Read the model definition and answer for the solid it produces. Units are mm, in the model's axes. A direction names the side the tool comes from. Round coordinates to 2 decimals unless told otherwise and drop trailing zeros. Write each loop counter-clockwise with the first axis right and the second up, starting at its lowest first coordinate (ties: lowest second). Pieces come first, ordered by that corner, then holes. Notation, with made-up numbers: (44, 22.25) - (57, 22.25) arc R26 ccw to (57, 54.25) - close; hole circle Ø4 at (73, 49). An arc over 180 degrees is marked (long way). One line per item, written item: value. Start each with the question number.
(1) A cutting plane is placed at D-D, the plane z = 3. Determine the outline of the cut face in (x, y), plus the area to 3 significant figures.
(2) Find the intervals of material crossed by L1, parallel to X at y = -24.4, z = 16.7 (3 decimals); L2, parallel to Y at x = 15, z = 4.5; L3, parallel to Y at x = -22, z = -16, in increasing order.
(3) A cutting plane is placed at C-C, the plane x = 0. Determine the outline of the cut face in (y, z) (1 decimal).
(4) A cutting plane is placed at B-B, the plane y = 15. Determine the outline of the cut face in (x, z).
(5) A cutting plane is placed at A-A, the plane z = -8.7. Determine the outline of the cut face in (x, y) (1 decimal), plus the area to 3 significant figures.
(6) For faces 1 (the face through (0, -23.13, 21)), 2 (the face through (0, -23.13, -13)), 3 (the face through (-0.55, 24.994, 3.944)), determine the directions among +Z, -Z, +X, -X, +Y, -Y from which every point of the face is accessible in a straight line to the end or side of a thin tool.
(7) The mould has two halves that part along Z. Classify faces 4 (the face through (-17, -4, 8)), 5 (the face through (25, -19, 4)), 6 (the face through (-19.08, -25.6, -6.36)): +Z half, -Z half, draft (parallel to the pull), parting line (faces both ways), or undercut.
(8) Flat-ended cylindrical pins translate along their axes: pin 1 Ø17 at (x, z) = (7, 15.5) entering from +Y; pin 2 Ø6 at (x, z) = (8.5, 19) entering from +Y; pin 3 Ø6 at (x, y) = (14.5, -2.5) entering from +Z. Find the tip coordinate at first contact, or state that the pin passes through.
Autodesk Inventor part; units mm, degrees
ref_plane "YZ Plane" through (0, 0, 0) normal (1, 0, 0) x (0, 1, 0)
ref_plane "XZ Plane" through (0, 0, 0) normal (0, 1, 0) x (-1, 0, 0)
ref_plane "XY Plane" through (0, 0, 0) normal (0, 0, 1) x (1, 0, 0)
sketch "Sketch1" plane through (0, 0, 0) normal (0, 0, 1) x (1, 0, 0)
  circle A0 centre (0, 0) radius 17
  arc A1 (25, 0) -> (-25, 0) centre (0, 0) ccw
  line L0 (-25, 0) -> (-25, -23.1305)
  line L1 (-25, -23.1305) -> (25, -23.1305)
  line L2 (25, -23.1305) -> (25, 0)
  circle A2 centre (-15, 15) radius 2.25
  circle A3 centre (15, 15) radius 2.25
  circle A4 centre (-15, -15) radius 2.25
  circle A5 centre (15, -15) radius 2.25
  dimension "d0" = 34
  dimension "d1" = 50
  dimension "d2" = 50
  dimension "d3" = 23.1305
  dimension "d54" = 4.5
  dimension "d57" = 30
  dimension "d60" = 30
  dimension "d63" = 15
  dimension "d64" = 15
extrude "Extrusion1" add sketch "Sketch1" along normal blind 8 contours L2 L1 L0 A1 | A2 | A3 | A4 | A5
sketch "Sketch2" plane through (-25, -23.1305, 0) normal (0, -1, 0) x (1, 0, 0)
  line L0 (0, 0) -> (50, 0) construction
  line L1 (0, 0) -> (0, 8)
  line L2 (0, -21.4) -> (50, -21.4)
  line L3 (50, -21.4) -> (50, 29.4)
  line L4 (50, 29.4) -> (0, 29.4)
  line L5 (0, 29.4) -> (0, -21.4)
  line L6 (0, -21.4) -> (50, 29.4) construction
  line L7 (50, -21.4) -> (0, 29.4) construction
  point P0 (25, 0)
  point P1 (25, 4)
  point P2 (25, 4)
  point P3 (0, 4)
  point P4 (25, 4)
  point P5 (25, 0)
  point P6 (50, 8)
  dimension "d7" = 50.8
  dimension "d65" = 50
  dimension "d66" = 50
extrude "Extrusion2" add sketch "Sketch2" along normal blind 5
sketch "Sketch3" plane through (-25, -28.1305, 0) normal (0, -1, 0) x (1, 0, 0)
  line L0 (50, 29.4) -> (0, 29.4)
  line L1 (0, 29.4) -> (0, -21.4)
  point P0 (25, 0)
  point P1 (8.0667, 16.7)
  point P2 (25, 16.7)
  point P3 (8.0667, -8.7)
  point P4 (25, -8.7)
  point P5 (41.9333, 16.7)
  point P6 (41.9333, -8.7)
  dimension "d39" = 16.9333
  dimension "d42" = 25.4
  dimension "d45" = 12.7
  dimension "d67" = 50
  dimension "d68" = 50.8
  dimension "d70" = 8.0667
hole "Hole2" at (-16.9333, -28.1305, 16.7) at (0, -28.1305, 16.7) at (-16.9333, -28.1305, -8.7) at (0, -28.1305, -8.7) at (16.9333, -28.1305, 16.7) at (16.9333, -28.1305, -8.7) direction (0, 1, 0) diameter 6.35 end through all
sketch "Sketch4" plane through (0, 0, 0) normal (0, 0, -1) x (-1, 0, 0)
  circle A0 centre (0, 0) radius 17
  line L0 (25, 0) -> (25, -23.1305)
  line L1 (25, -23.1305) -> (-25, -23.1305)
  point P0 (-15, 15)
  point P1 (15, 15)
  point P2 (-15, -15)
  point P3 (15, -15)
  dimension "d80" = 30
  dimension "d83" = 30
  dimension "d86" = 15
  dimension "d87" = 15
hole "Hole3" at (15, 15, 0) at (-15, 15, 0) at (15, -15, 0) at (-15, -15, 0) direction (0, 0, 1) diameter 4.5 end through all
equation "\"d2\" = d1"
equation "\"d65\" = d66"
properties part number "ff12_mount"
Here are the results:
1. outline: (-25, -28.13) - (25, -28.13) - (25, 0) arc R25 ccw to (-25, 0) - close; hole circle Ø4.5 at (-15, -15); hole circle Ø4.5 at (-15, 15); hole circle Ø34 at (0, 0); hole circle Ø4.5 at (15, -15); hole circle Ø4.5 at (15, 15)
1. area: 1,420 mm²
2. L1: -25 to -20.108, -13.758 to -3.175, 3.175 to 13.758, 20.108 to 25
2. L2: -28.13 to -17.25, -12.75 to -8, 8 to 12.75, 17.25 to 20
2. L3: -28.13 to -23.13
3. outline: (-28.1, -21.4) - (-23.1, -21.4) - (-23.1, -11.9) - (-28.1, -11.9) - close; (-28.1, -5.5) - (-23.1, -5.5) - (-23.1, 0) - (-17, 0) - (-17, 8) - (-23.1, 8) - (-23.1, 13.5) - (-28.1, 13.5) - close; (-28.1, 19.9) - (-23.1, 19.9) - (-23.1, 29.4) - (-28.1, 29.4) - close; (17, 0) - (25, 0) - (25, 8) - (17, 8) - close
4. outline: (-20, 0) - (-17.25, 0) - (-17.25, 8) - (-20, 8) - close; (-12.75, 0) - (-8, 0) - (-8, 8) - (-12.75, 8) - close; (8, 0) - (12.75, 0) - (12.75, 8) - (8, 8) - close; (17.25, 0) - (20, 0) - (20, 8) - (17.25, 8) - close
5. outline: (-25, -28.1) - (-20.1, -28.1) - (-20.1, -23.1) - (-25, -23.1) - close; (-13.8, -28.1) - (-3.2, -28.1) - (-3.2, -23.1) - (-13.8, -23.1) - close; (3.2, -28.1) - (13.8, -28.1) - (13.8, -23.1) - (3.2, -23.1) - close; (20.1, -28.1) - (25, -28.1) - (25, -23.1) - (20.1, -23.1) - close
5. area: 155 mm²
6. face 1: +Z, +X, -X, +Y
6. face 2: -Z, +X, -X, +Y
6. face 3: +Z, -Z, +Y
7. face 4: +Z half
7. face 5: draft
7. face 6: undercut
8. pin 1: y = 24.82
8. pin 2: y = -23.13
8. pin 3: z = 8
